from build123d import *

# Parameters (mm, degrees)
SKETCH1_R            = 2.2
BOSS_EXTRUDE1_DEPTH  = 65
CUT_EXTRUDE1_DEPTH   = 4.1
FILLET1_R            = 0.5
FILLET1_OF_MIRROR1_R = 0.5
SKETCH4_W            = 30
SKETCH4_H            = 40
CUT_EXTRUDE2_DEPTH   = 82.688432474
FILLET2_R            = 4


with BuildPart() as part:
    # Sketch1 → Boss-Extrude1 (new body)
    with BuildSketch(Plane(origin=(0, 0, 0), x_dir=(1, 0, 0), z_dir=(0, 1, 0))):
        with BuildLine():
            Line((0, 6), (42, 6))
            ThreePointArc((42, 6), (48, 0), (42, -6))
            Line((42, -6), (0, -6))
            ThreePointArc((0, -6), (-6, 0), (0, 6))
        make_face()
        with Locations(Location((0, 0, 0), (0, 0, 270))):
            Circle(SKETCH1_R, mode=Mode.SUBTRACT)
        with Locations(Location((42, 0, 0), (0, 0, 270))):
            Circle(SKETCH1_R, mode=Mode.SUBTRACT)
    extrude(amount=BOSS_EXTRUDE1_DEPTH)

    # Sketch3 → Cut-Extrude1 (cut)
    with BuildSketch(Plane(origin=(0, 61, 0), x_dir=(1, 0, 0), z_dir=(0, 1, 0))):
        Polygon((4.099186911, 0), (2.049593456, 3.55), (-9.046065911, 3.55), (-8.518024666, -3.55), (2.049593456, -3.55), align=None)
        Polygon((39.950406544, 3.55), (51.046065911, 3.55), (50.518024666, -3.55), (39.950406544, -3.55), (37.900813089, 0), align=None)
    cut_extrude1 = extrude(amount=-CUT_EXTRUDE1_DEPTH, mode=Mode.SUBTRACT)

    # Fillet1
    fillet1_edges = [part.edges().sort_by_distance(p)[0] for p in [
        (46.837096236, 58.95, 3.55),
        (46.837096236, 58.95, -3.55),
        (-4.837096236, 58.95, -3.55),
        (-4.837096236, 58.95, 3.55),
    ]]
    fillet(fillet1_edges, radius=FILLET1_R)

    # Mirror1: Cut-Extrude1 across plane
    add(cut_extrude1.mirror(Plane.ZX.offset(32.5)), mode=Mode.SUBTRACT)

    # Fillet1 of Mirror1
    fillet1_of_mirror1_edges = [part.edges().sort_by_distance(p)[0] for p in [
        (46.837096236, 6.05, 3.55),
        (46.837096236, 6.05, -3.55),
        (-4.837096236, 6.05, -3.55),
        (-4.837096236, 6.05, 3.55),
    ]]
    fillet(fillet1_of_mirror1_edges, radius=FILLET1_OF_MIRROR1_R)

    # Sketch4 → Cut-Extrude2 (cut, through all)
    with BuildSketch(Plane(origin=(0, 0, -6), x_dir=(-1, 0, 0), z_dir=(0, 0, -1))):
        with Locations((-21, 32.5)):
            Rectangle(SKETCH4_W, SKETCH4_H)
    extrude(amount=-CUT_EXTRUDE2_DEPTH, mode=Mode.SUBTRACT)

    # Fillet2
    fillet2_edges = [part.edges().sort_by_distance(p)[0] for p in [
        (6, 52.5, 0),
        (6, 12.5, 0),
        (36, 12.5, 0),
        (36, 52.5, 0),
    ]]
    fillet(fillet2_edges, radius=FILLET2_R)


solid = part.part
For this review, take the finished solid that the model builds, in its own axes (mm). A direction names the side the tool comes from. Round coordinates to 2 decimals unless told otherwise and drop trailing zeros. Write each loop counter-clockwise with the first axis right and the second up, starting at its lowest first coordinate (ties: lowest second). Pieces come first, ordered by that corner, then holes. Notation, with made-up numbers: (59.25, 32.5) -> (98.25, 32.5) arc R13 ccw to (98.25, 50.5) -> close; hole circle Ø1 at (-26, -4.5). An arc over 180 degrees is marked (long way). Use CSV: the item, a comma, the result in double quotes.
(1) Consider section B-B, the plane x = 31. Give the boundary of the cut face in (y, z).
Computed values:
outline,"(0, -6) -> (12.5, -6) -> (12.5, 6) -> (0, 6) -> close; (52.5, -6) -> (65, -6) -> (65, 6) -> (52.5, 6) -> close"
(2) Consider section C-C, the plane y = 9.5. Give the boundary of the cut face in (x, z), plus the area to 3 significant figures.
Computed values:
outline,"(0, -6) -> (42, -6) arc R6 ccw to (42, 6) -> (0, 6) arc R6 ccw to start; hole circle Ø4.4 at (0, 0); hole circle Ø4.4 at (42, 0)"
area,"587 mm²"
(3) For faces 4 (the face through (34.797, 51.359, 0.084)), 5 (the face through (3.06, 58.98, 1.8)), 6 (the face through (38.94, 58.98, 1.8)), list the 3-axis set-ups (+Z, -Z, +X, -X, +Y, -Y) from which the entire face can be reached by the end or side of a thin tool; tool diameter is ignored.
Computed values:
face 4,"+Z, -Z"
face 5,"-X"
face 6,"+X"
(4) Draft analysis for pull direction Y (two halves, no side actions). For faces 1 (the face through (38.91, 6.02, -1.75)), 2 (the face through (39.852, 62.972, -0.477)), 3 (the face through (21, 0, 0)), state which applies: +Y half, -Y half, draft (parallel to the pull), parting line (faces both ways), or undercut.
Computed values:
face 1,"undercut"
face 2,"draft"
face 3,"-Y half"
(5) Consider section D-D, the plane y = 50. Give the boundary of the cut face in (x, z).
Computed values:
outline,"(0, -6) -> (6.29, -6) -> (6.29, 6) -> (0, 6) arc R6 ccw to start; (35.71, -6) -> (42, -6) arc R6 ccw to (42, 6) -> (35.71, 6) -> close; hole circle Ø4.4 at (0, 0); hole circle Ø4.4 at (42, 0)"
(6) To check wall thickness, follow L1, parallel to Y at x = 43.5, z = -2.75; L2, parallel to X at y = 1.8, z = 0; L3, parallel to Y at x = 23, z = 0. State the ranges of each line that lie inside material, in increasing order. Write a range as [from, to].
Computed values:
L1,"[0, 4], [8.1, 56.9], [61, 65]"
L2,"[-6, -2.2], [2.2, 39.8], [44.2, 48]"
L3,"[0, 12.5], [52.5, 65]"
(7) Consider section A-A, the plane y = 18. Give the boundary of the cut face in (x, z), plus the area to 3 significant figures.
Computed values:
outline,"(0, -6) -> (6, -6) -> (6, 6) -> (0, 6) arc R6 ccw to start; (36, -6) -> (42, -6) arc R6 ccw to (42, 6) -> (36, 6) -> close; hole circle Ø4.4 at (0, 0); hole circle Ø4.4 at (42, 0)"
area,"227 mm²"
(8) Clearance check with flat-ended pins moving along their axes: P1, Ø2.5, axis at x = 0, z = 0, coming from the -Y side; P2, Ø1.2, axis at x = 43.5, y = 59, coming from the -Z side. State where each tip first meets the part, or that it passes through.
Computed values:
P1,"through"
P2,"z = -5.93"
